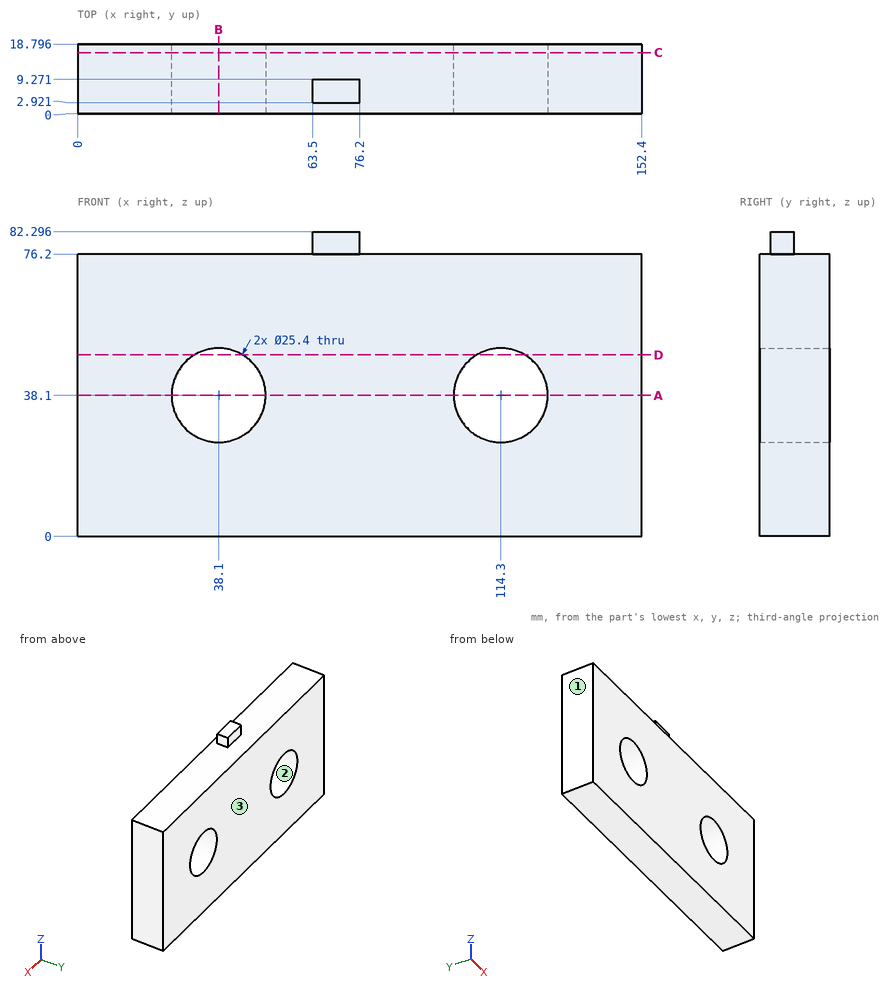
Source: three-view drawing plus pictorial views. Frame: mm from the lowest corner of the part. Coordinates: 2 decimals unless noted, no trailing zeros. Loops run counter-clockwise (first coordinate to the right, second up) from the corner with the lowest first, then second, coordinate; pieces in that order, holes last. Notation, with made-up numbers: (-17, 53.25) -> (37, 53.25) arc R17 ccw to (37, 86.25) -> close; hole circle Ø1 at (11, 66). An arc over 180 degrees is marked (long way). Answer in a Markdown table with one row per item. Add a question column.
Q1. Section D-D on z = 49. Return the cut outline in (x, y).
Q2. Pull-direction query (X, two-part tool) for the marked faces 1, 2 and 3; classes: pulls with the +X half, pulls with the -X half, needs draft (parallel to the pull), parting line crosses it, or undercut.
Q3. Section A-A on z = 38.1. Return the cut outline in (x, y), and give its area (3 significant figures).
Q4. Section B-B on x = 38.1. Return the cut outline in (y, z).
Q5. Ray query, line 1 along Z through (x, y) = (38.1, 7.25); line 2 along X through (y, z) = (14.25, 41.5); line 3 along Z through (x, y) = (122.5, 16). Return the intervals inside material, ascending.
Q6. Section C-C on y = 16.5. Return the cut outline in (x, z), and give its area (3 significant figures).
Q7. Contact query for flat-ended pins moving along their axis: pin 1 Ø3 at (x, z) = (67.5, 79) entering from -Y; pin 2 Ø4 at (x, y) = (135, 16) entering from +Z; pin 3 Ø3 at (x, z) = (71, 79.5) entering from +Y. Output: stop coordinate, or through.
Computed values:
| question | item | result |
|---|---|---|
| 1 | outline | (0, 0) -> (31.58, 0) -> (31.58, 18.8) -> (0, 18.8) -> close; (44.62, 0) -> (107.78, 0) -> (107.78, 18.8) -> (44.62, 18.8) -> close; (120.82, 0) -> (152.4, 0) -> (152.4, 18.8) -> (120.82, 18.8) -> close |
| 2 | face 1 | pulls with the -X half |
| 2 | face 2 | undercut |
| 2 | face 3 | needs draft |
| 3 | outline | (0, 0) -> (25.4, 0) -> (25.4, 18.8) -> (0, 18.8) -> close; (50.8, 0) -> (101.6, 0) -> (101.6, 18.8) -> (50.8, 18.8) -> close; (127, 0) -> (152.4, 0) -> (152.4, 18.8) -> (127, 18.8) -> close |
| 3 | area | 1,910 mm^2 |
| 4 | outline | (0, 0) -> (18.8, 0) -> (18.8, 25.4) -> (0, 25.4) -> close; (0, 50.8) -> (18.8, 50.8) -> (18.8, 76.2) -> (0, 76.2) -> close |
| 5 | line 1 | z = 0 to 25.4, 50.8 to 76.2 |
| 5 | line 2 | x = 0 to 25.86, 50.34 to 102.06, 126.54 to 152.4 |
| 5 | line 3 | z = 0 to 28.4, 47.8 to 76.2 |
| 6 | outline | (0, 0) -> (152.4, 0) -> (152.4, 76.2) -> (0, 76.2) -> close; hole circle Ø25.4 at (38.1, 38.1); hole circle Ø25.4 at (114.3, 38.1) |
| 6 | area | 10,600 mm^2 |
| 7 | pin 1 | stops at y = 2.92 |
| 7 | pin 2 | stops at z = 76.2 |
| 7 | pin 3 | stops at y = 9.27 |
